CAD build for the part. Positions are in the model's coordinates, mm. A direction names the side the tool comes from. Round coordinates to 2 decimals unless told otherwise and drop trailing zeros. Order: outer loops, then holes, each group sorted by start corner. A loop starts at its lowest first (then second) coordinate and runs counter-clockwise, first axis right, second up. Notation, with made-up numbers: M 31.25,-8 L 62.25,-8 A16 cw 62.25,20 Z; hole C -36,14.25 d7. An arc over 180 degrees is marked long. Put each result on its own line as item: value.
```python
from build123d import *

# Parameters (mm, degrees)
CORTAR_EXTRUIR2_DEPTH = 5


with BuildPart() as part:
    # Croquis1 → Revolución1 (revolve)
    with BuildSketch(Plane(origin=(0, 0, 0), x_dir=(1, 0, 0), z_dir=(0, 1, 0)), mode=Mode.PRIVATE) as revoluci_n1_sk:
        Polygon((0, 0), (49.556624327, 0), (51, 2.5), (58, 2.5), (58, 3), (59.5, 3), (60, 3.5), (60, 5), (59.5, 5.5), (36.5, 5.5), (36.5, 3), (0, 3), align=None)
    revolve(revoluci_n1_sk.sketch.rotate(Axis((0, 0, 0), (1, 0, 0)), 180), axis=Axis((0, 0, 0), (1, 0, 0)))

    # Croquis3 → Cortar-Extruir2 (cut)
    with BuildSketch(Plane(origin=(60, 0, 0), x_dir=(0, 0, -1), z_dir=(1, 0, 0))):
        Polygon((3.484172317, -0.332480476), (2.030022697, 2.8511415), (-1.45414962, 3.183621975), (-3.484172317, 0.332480476), (-2.030022697, -2.8511415), (1.45414962, -3.183621975), align=None)
    extrude(amount=-CORTAR_EXTRUIR2_DEPTH, mode=Mode.SUBTRACT)


solid = part.part
```
Item 1: Mould opens along Z. For faces 1 (the flat face through (57.535, 1.778, 2.455)), 2 (the cylindrical face through (17.99, -0.9, 2.86)), 3 (the flat face through (57.535, -3.015, 0.312)), 4 (the flat face through (36.5, 2.4, 2.4)) say: pulls with the +Z half, pulls with the -Z half, needs draft (parallel to the pull), parting line crosses it, or undercut.
Answers below:
face 1: undercut
face 2: parting line crosses it
face 3: undercut
face 4: needs draft
Item 2: Tool access for faces 5 (the flat face through (60, 3.3, -2.2)), 6 (the flat face through (57.535, -1.237, 2.767)): list every direction of +Z, -Z, +X, -X, +Y, -Y with a clear straight run to the whole face (end or side of a thin tool).
Answers below:
face 5: +Z, -Z, +X, +Y, -Y
face 6: +X
Item 3: Band-saw the part on B-B on x = 32. Give the cut face in (y, z), and give its area (3 significant figures).
Answers below:
outline: C 0,0 d6
area: 28.3 mm²
Item 4: Band-saw the part on A-A on x = 52. Give the cut face in (y, z), and give its area (3 significant figures).
Answers below:
outline: C 0,0 d11; hole C 0,0 d5
area: 75.4 mm²
Item 5: Probe line 1 along Y through (x, z) = (52.15, 0); line 2 along X through (y, z) = (-3.75, 0.25); line 3 along X through (y, z) = (0, 0). List the from-to ranges inside material, lowest first. Write a range as [from, to].
Answers below:
line 1: [-5.5, -2.5], [2.5, 5.5]
line 2: [36.5, 60]
line 3: [0, 49.56]
Item 6: Pin check, flat tips, straight feed: P1, Ø1, axis at x = 7.5, y = -2, coming from the -Z side; P2, Ø1.5, axis at x = 54, y = -1, coming from the +Z side; P3, Ø4, axis at x = 36.5, z = 4, coming from the -Y side. Stop position of each tip, or through.
Answers below:
P1: z = -2.6
P2: z = 5.49
P3: y = -5.12
